Autodesk Inventor part; units mm, degrees
ref_plane "YZ Plane" through (0, 0, 0) normal (1, 0, 0) x (0, 1, 0)
ref_plane "XZ Plane" through (0, 0, 0) normal (0, 1, 0) x (-1, 0, 0)
ref_plane "XY Plane" through (0, 0, 0) normal (0, 0, 1) x (1, 0, 0)
sketch "Sketch1" plane through (0, 0, 0) normal (0, 1, 0) x (-1, 0, 0)
  line L0 (-40.64, 58.42) -> (40.64, 58.42)
  line L1 (40.64, 58.42) -> (40.64, -58.42)
  line L2 (40.64, -58.42) -> (-40.64, -58.42)
  line L3 (-40.64, -58.42) -> (-40.64, 58.42)
  point P0 (0, 0)
  point P1 (0, 58.42)
  point P2 (40.64, 0)
  dimension "d0" = 81.28
  dimension "d1" = 116.84
extrude "Extrusion1" add sketch "Sketch1" along normal blind 12.7
fillet "Fillet1" radius 12.7 4 edges at (-40.64, 6.35, 58.42) (-40.64, 6.35, -58.42) (40.64, 6.35, 58.42) (40.64, 6.35, -58.42)
sketch "Sketch2" plane through (0, 12.7, 0) normal (0, 1, 0) x (1, 0, 0)
  arc A0 (-27.94, 58.42) -> (-40.64, 45.72) centre (-27.94, 45.72) ccw
  point P0 (0, 0)
hole "Hole1" at (-27.94, 12.7, -45.72) direction (0, -1, 0) diameter 6.7564 end through all countersink diameter 12.8778 countersink angle 82
sketch "Sketch3" plane through (0, 12.7, 0) normal (0, 1, 0) x (1, 0, 0)
  arc A0 (-40.64, -45.72) -> (-27.94, -58.42) centre (-27.94, -45.72) ccw
  point P0 (0, 0)
hole "Hole2" at (-27.94, 12.7, 45.72) direction (0, -1, 0) diameter 6.7564 end through all countersink diameter 12.8778 countersink angle 82
sketch "Sketch4" plane through (0, 12.7, 0) normal (0, 1, 0) x (1, 0, 0)
  arc A0 (27.94, -58.42) -> (40.64, -45.72) centre (27.94, -45.72) ccw
  point P0 (0, 0)
hole "Hole3" at (27.94, 12.7, 45.72) direction (0, -1, 0) diameter 6.7564 end through all countersink diameter 12.8778 countersink angle 82
sketch "Sketch5" plane through (0, 12.7, 0) normal (0, 1, 0) x (1, 0, 0)
  arc A0 (40.64, 45.72) -> (27.94, 58.42) centre (27.94, 45.72) ccw
  point P0 (0, 0)
hole "Hole4" at (27.94, 12.7, -45.72) direction (0, -1, 0) diameter 6.7564 end through all countersink diameter 12.8778 countersink angle 82
properties part number "Base plate"
Could you check a few things on this model? Use its own coordinates, in mm. Give positions to 0.01 mm unless a question says otherwise; leave off trailing zeros. Order: outer loops, then holes, each group sorted by start corner. A loop starts at its lowest first (then second) coordinate and runs counter-clockwise, first axis right, second up.
1. We'd pull the mould along X, two halves only. Please class faces 1 (the cylindrical face through (-30.789, 4.525, -43.904)), 2 (the cylindrical face through (37.02, 6.44, -54.6)), 3 (the cylindrical face through (-36.82, 6.44, -54.8)): pulls with the +X half, pulls with the -X half, needs draft (parallel to the pull), parting line crosses it, or undercut.
2. Will these pins go through, and if not, where does the flat tip stop? P1, Ø11, axis at x = -27.94, z = 45.72, coming from the +Y side; P2, Ø6, axis at x = 27.94, z = 45.72, coming from the +Y side; P3, Ø8, axis at x = 27.94, z = -45.72, coming from the +Y side.
3. I need wall thicknesses on L1, parallel to X at y = 5, z = 45.72; L2, parallel to Z at x = 27.94, y = 5.75; L3, parallel to X at y = 3, z = 47.5. Which ranges of each line are inside material? Lowest first, please.
4. Suppose I cut it at A-A (y = 2.5). List the corners of the cut face in (x, z) for me.
Solved:
1. face 1: undercut
1. face 2: pulls with the +X half
1. face 3: pulls with the -X half
2. P1: stops at y = 11.62
2. P2: passes through
2. P3: stops at y = 9.89
3. L1: x = -40.64 to -31.32, -24.56 to 24.56, 31.32 to 40.64
3. L2: z = -58.42 to -49.1, -42.34 to 42.34, 49.1 to 58.42
3. L3: x = -40.51 to -30.81, -25.07 to 25.07, 30.81 to 40.51
4. outline: (-40.64, -45.72) arc R12.7 ccw to (-27.94, -58.42) - (27.94, -58.42) arc R12.7 ccw to (40.64, -45.72) - (40.64, 45.72) arc R12.7 ccw to (27.94, 58.42) - (-27.94, 58.42) arc R12.7 ccw to (-40.64, 45.72) - close; hole circle Ø6.76 at (-27.94, -45.72); hole circle Ø6.76 at (-27.94, 45.72); hole circle Ø6.76 at (27.94, -45.72); hole circle Ø6.76 at (27.94, 45.72)
